from build123d import *

# Parameters (mm, degrees)
SKETCH3_R           = 3.5
SKETCH3_R_2         = 2.5
BOSS_EXTRUDE3_DEPTH = 2
SKETCH4_R           = 2.75
SKETCH4_R_2         = 1.65
BOSS_EXTRUDE4_DEPTH = 4
SKETCH5_R           = 2.5
CUT_EXTRUDE1_DEPTH  = 2


with BuildPart() as part:
    # Sketch3 → Boss-Extrude3 (new body)
    with BuildSketch(Plane(origin=(0, 0, 0), x_dir=(1, 0, 0), z_dir=(0, 1, 0))):
        with Locations(Location((0, 0, 0), (0, 0, 270))):
            Circle(SKETCH3_R)
        with Locations(Location((0, 0, 0), (0, 0, 270))):
            Circle(SKETCH3_R_2, mode=Mode.SUBTRACT)
    extrude(amount=BOSS_EXTRUDE3_DEPTH)

    # Sketch4 → Boss-Extrude4 (add)
    with BuildSketch(Plane(origin=(0, 2, 0), x_dir=(1, 0, 0), z_dir=(0, 1, 0))):
        with Locations(Location((0, 0, 0), (0, 0, 270))):
            Circle(SKETCH4_R)
        with Locations(Location((0, 0, 0), (0, 0, 270))):
            Circle(SKETCH4_R_2, mode=Mode.SUBTRACT)
    extrude(amount=BOSS_EXTRUDE4_DEPTH)

    # Sketch5 → Cut-Extrude1 (cut)
    with BuildSketch(Plane.XZ.offset(-2)):
        with Locations(Location((0, 0, 0), (0, 0, 270))):
            Circle(SKETCH5_R)
    extrude(amount=-CUT_EXTRUDE1_DEPTH, mode=Mode.SUBTRACT)


solid = part.part
The model under review builds one solid part; all positions refer to its coordinate system, in mm. A direction names the side the tool comes from. Give positions to 0.01 mm unless a question says otherwise; leave off trailing zeros. Order: outer loops, then holes, each group sorted by start corner. A loop starts at its lowest first (then second) coordinate and runs counter-clockwise, first axis right, second up. Notation, with made-up numbers: M 5,82 L 52,82 A22 cw 52,121 Z; hole C 44.25,86.5 d9. An arc over 180 degrees is marked long. Answer in a Markdown table with one row per item. Add a question column.
1. Add section B-B on x = 0. State the section outline as (y, z) points, plus the area to 3 significant figures.
2. Mouldability with a two-part tool opening along X and no side actions: class faces 1 (the flat face through (0, 6, 2)), 2 (the cylindrical face through (-2.685, 3.972, -0.596)), 3 (the cylindrical face through (-1, 4.99, -1.31)) as released by +X, released by -X, zero draft, split by the parting line, or undercut.
3. Add section D-D on z = 2.25. State the section outline as (x, y) points, plus the area to 3 significant figures.
4. To check wall thickness, follow line 1 along X through (y, z) = (2.65, 0); line 2 along X through (y, z) = (0.5, 0); line 3 along Z through (x, y) = (-0.75, 1). State the ranges of each line that lie inside material, in increasing order.
5. Machinability: for faces 4 (the cylindrical face through (-3.417, 0.986, -0.759)), 5 (the flat face through (-1, 2, -3)), 6 (the flat face through (-1, 4, -2)), which of the approach directions +Z, -Z, +X, -X, +Y, -Y give a long, thin tool a straight path to every point of the face, cutting with its end or side? Answer none if there is none.
6. Add section C-C on y = 0.8. State the section outline as (x, z) points, plus the area to 3 significant figures.
7. Add section A-A on z = 0. State the section outline as (x, y) points, plus the area to 3 significant figures.
8. For pin 1 Ø1.5 at (y, z) = (2, 2.5) entering from -X; pin 2 Ø1 at (x, y) = (2, 4) entering from -Z; pin 3 Ø1.5 at (x, y) = (-1, 1) entering from -Z, all flat-tipped, find the tip position at first contact; note any pin that passes through.
The answers:
| question | item | result |
|---|---|---|
| 1 | outline | M 0,-3.5 L 2,-3.5 L 2,-2.75 L 6,-2.75 L 6,-1.65 L 4,-1.65 L 4,-2.5 L 0,-2.5 Z; M 0,2.5 L 4,2.5 L 4,1.65 L 6,1.65 L 6,2.75 L 2,2.75 L 2,3.5 L 0,3.5 Z |
| 1 | area | 9.40 mm2 |
| 2 | face 1 | zero draft |
| 2 | face 2 | split by the parting line |
| 2 | face 3 | undercut |
| 3 | outline | M -2.68,0 L -1.09,0 L -1.09,4 L 1.09,4 L 1.09,0 L 2.68,0 L 2.68,2 L 1.58,2 L 1.58,6 L -1.58,6 L -1.58,2 L -2.68,2 Z |
| 3 | area | 14.7 mm2 |
| 4 | line 1 | -2.75 to -2.5, 2.5 to 2.75 |
| 4 | line 2 | -3.5 to -2.5, 2.5 to 3.5 |
| 4 | line 3 | -3.42 to -2.38, 2.38 to 3.42 |
| 5 | face 4 | +Y, -Y |
| 5 | face 5 | +Y |
| 5 | face 6 | -Y |
| 6 | outline | C 0,0 d7; hole C 0,0 d5 |
| 6 | area | 18.8 mm2 |
| 7 | outline | M -3.5,0 L -2.5,0 L -2.5,4 L -1.65,4 L -1.65,6 L -2.75,6 L -2.75,2 L -3.5,2 Z; M 1.65,4 L 2.5,4 L 2.5,0 L 3.5,0 L 3.5,2 L 2.75,2 L 2.75,6 L 1.65,6 Z |
| 7 | area | 9.40 mm2 |
| 8 | pin 1 | x = -3.03 |
| 8 | pin 2 | z = -2.3 |
| 8 | pin 3 | z = -3.49 |
